Verification items for the finished model (mm, model axes). Face numbers are marked on the shaded views. A direction names the side the tool comes from. Coordinates: 2 decimals unless noted, no trailing zeros. Order: outer loops, then holes, each group sorted by start corner. A loop starts at its lowest first (then second) coordinate and runs counter-clockwise, first axis right, second up. Notation, with made-up numbers: M -8.5,12 L 3.5,12 A16 cw 3.5,38 Z; hole C -5.5,76 d10. An arc over 180 degrees is marked long. Return JSON: item names as keys, results as strings. Group by question number.
Q1. Section check B-B, the plane z = 3.5. Enter the section's corners in (x, y).
Q2. Thickness scan on probe 1 along X at (y, z) = (0, -8.2); probe 2 along X at (y, z) = (0, -8.4); probe 3 along Y at (x, z) = (0, -7.95). Record the ranges inside material, lowest first.
Q3. Go/stop test with flat-tipped pins: pin 1 Ø1.4 at (y, z) = (-1, -9) entering from -X; pin 2 Ø1 at (x, z) = (-2, 9) entering from +Y; pin 3 Ø1.5 at (x, y) = (-0.5, 0.5) entering from +Z. Record where each tip stops, or that it passes through.
Q4. Access from +Z, -Z, +X, -X, +Y, -Y to the whole of each face (thin tool, end or side, straight path). Record for the marked faces 5, 6 and 7.
Q5. Section check C-C, the plane y = 0. Enter the section's corners in (x, z).
Q6. Section check A-A, the plane x = -3. Enter the section's corners in (y, z).
Q7. Section check D-D, the plane z = 0. Enter the section's corners in (x, y), then the cut area to 3 significant figures.
Q8. Mould release check, pull along Y, two halves, no side actions. Record for the marked faces 1, 2, 3 and 4: pulls with the +Y half, pulls with the -Y half, needs draft (parallel to the pull), parting line crosses it, or undercut.
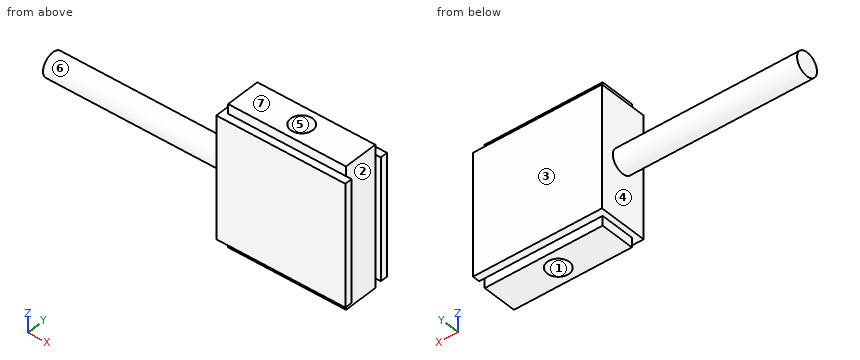
from build123d import *

# Parameters (mm, degrees)
F0_W      = 16
F0_H      = 19.1
F1_DEPTH  = 2.35
F2_W      = 17.5
F2_H      = 16.5
F3_DEPTH  = 1
F4_DEPTH  = 2.35
F6_R      = 1.6
F7_DEPTH  = 25
F8_R      = 1.5
F9_DEPTH  = 2.8
F10_R     = 1.5
F11_DEPTH = 2.8


with BuildPart() as f1:
    # F0 (on Front) → F1 (new body)
    with BuildSketch(Plane.XZ):
        Rectangle(F0_W, F0_H)
    extrude(amount=F1_DEPTH)

    # F2 (on face) → F3 (join)
    with BuildSketch(Plane.XZ.offset(2.35)):
        Rectangle(F2_W, F2_H)
    extrude(amount=F3_DEPTH)

    # F4 (add, through all): a face of the model
    f4_faces = [f1.faces().sort_by_distance(p)[0] for p in [
        (-8.375, -2.35, 0),
    ]]
    extrude(f4_faces, amount=F4_DEPTH)

    # F5: F1 across plane


with BuildPart() as f1_1:
    add(f1.part)
    add(f1.part.mirror(Plane.XZ))

    # F6 (on face) → F7 (join)
    with BuildSketch(Plane(origin=(-8.75, 0, 0), x_dir=(0, -1, 0), z_dir=(-1, 0, 0))):
        Circle(F6_R)
    extrude(amount=F7_DEPTH)

    # F8 (on face) → F9 (cut)
    with BuildSketch(Plane.XY.offset(9.55)):
        Circle(F8_R)
    extrude(amount=-F9_DEPTH, mode=Mode.SUBTRACT)

    # F10 (on face) → F11 (cut)
    with BuildSketch(Plane(origin=(0, 0, -9.55), x_dir=(1, 0, 0), z_dir=(0, 0, -1))):
        Circle(F10_R)
    extrude(amount=-F11_DEPTH, mode=Mode.SUBTRACT)


solid = f1_1.part
Numbers:
{
 "1": {"outline": "M -8.75,-3.35 L 8.75,-3.35 L 8.75,-2.35 L 8,-2.35 L 8,2.35 L 8.75,2.35 L 8.75,3.35 L -8.75,3.35 Z"},
 "2": {"probe 1": "x = -8.75 to -1.5, 1.5 to 8", "probe 2": "x = -8 to -1.5, 1.5 to 8", "probe 3": "y = -3.35 to -1.5, 1.5 to 3.35"},
 "3": {"pin 1": "stops at x = -8", "pin 2": "stops at y = 2.35", "pin 3": "stops at z = 6.75"},
 "4": {"face 5": "+Z", "face 6": "-X", "face 7": "+Z, +X, -X, +Y, -Y"},
 "5": {"outline": "M -33.75,-1.6 L -8.75,-1.6 L -8.75,-8.25 L -8,-8.25 L -8,-9.55 L -1.5,-9.55 L -1.5,-6.75 L 1.5,-6.75 L 1.5,-9.55 L 8,-9.55 L 8,9.55 L 1.5,9.55 L 1.5,6.75 L -1.5,6.75 L -1.5,9.55 L -8,9.55 L -8,8.25 L -8.75,8.25 L -8.75,1.6 L -33.75,1.6 Z"},
 "6": {"outline": "M -3.35,-8.25 L -2.35,-8.25 L -2.35,-9.55 L 2.35,-9.55 L 2.35,-8.25 L 3.35,-8.25 L 3.35,8.25 L 2.35,8.25 L 2.35,9.55 L -2.35,9.55 L -2.35,8.25 L -3.35,8.25 Z"},
 "7": {"outline": "M -33.75,-1.6 L -8.75,-1.6 L -8.75,-3.35 L 8.75,-3.35 L 8.75,-2.35 L 8,-2.35 L 8,2.35 L 8.75,2.35 L 8.75,3.35 L -8.75,3.35 L -8.75,1.6 L -33.75,1.6 Z", "area": "194 mm2"},
 "8": {"face 1": "undercut", "face 2": "undercut", "face 3": "pulls with the +Y half", "face 4": "needs draft"}
}
